The model under review builds one solid part; all positions refer to its coordinate system, in mm. Face numbers are marked on the shaded views. Coordinates: 2 decimals unless noted, no trailing zeros. Loops run counter-clockwise (first coordinate to the right, second up) from the corner with the lowest first, then second, coordinate; pieces in that order, holes last. Notation, with made-up numbers: (43.5, 7) - (99.5, 7) arc R15 cw to (99.5, 19) - close; hole circle Ø10 at (88, 62.25). An arc over 180 degrees is marked (long way). Use a Markdown table: item, result. Add a question column.
1) The part is to be moulded in two halves that separate along X. For the marked faces 1, 2 and 3, say which applies: pulls with the +X half, pulls with the -X half, needs draft (parallel to the pull), parting line crosses it, or undercut.
2) Add section C-C, the plane x = 0. Give the boundary of the cut face in (y, z).
3) Clearance check with flat-ended pins moving along their axes: pin 1 (3 mm diameter, centred on y = -54, z = 26.5, fed in from -X); pin 2 (21.5 mm diameter, centred on y = -37, z = 8, fed in from -X); pin 3 (6.5 mm diameter, centred on x = -6.5, z = 2, fed in from -Y). State where each tip first meets the part, or that it passes through.
4) Add section B-B, the plane z = 1.5. Give the boundary of the cut face in (x, y), and give its area (3 significant figures).
5) Add section D-D, the plane z = 23.5. Give the boundary of the cut face in (x, y), and give its area (3 significant figures).
6) To check wall thickness, follow L1, parallel to X at y = -8, z = -3; L2, parallel to X at y = -95, z = -3.5; L3, parallel to Z at x = 35, y = -8. State the ranges of each line that lie inside material, in increasing order. Write a range as [from, to].
7) Add section A-A, the plane y = -25.5. Give the boundary of the cut face in (x, z), and give its area (3 significant figures).
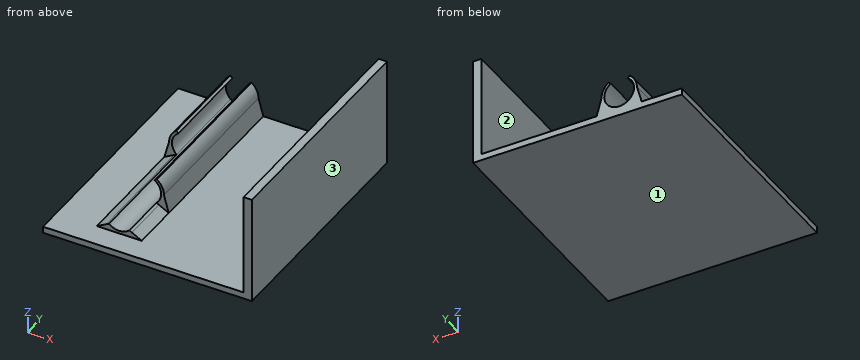
```python
from build123d import *

# Parameters (mm, degrees)
F1_DEPTH = 90
F2_DEPTH = 40
F0_W     = 3.4774128616
F0_H     = 42.5927758359
F3_DEPTH = 100
F4_DEPTH = 70


# Not quite as in the source:
# - a feature names something its author has since deleted; it is built from what else it names


with BuildPart() as f1:
    # F0 (on Front) → F1 (new body)
    with BuildSketch(Plane.XZ):
        with BuildLine():
            ThreePointArc((4.2720749172, -4.5620034965), (0, -6.25), (-4.2720749172, -4.5620034965))
            Line((-4.2720749172, -4.5620034965), (-5.3278356976, -5.1455675625))
            ThreePointArc((-5.3278356976, -5.1455675625), (-2.8939428024, -6.818195789), (0, -7.4069358551))
            ThreePointArc((0, -7.4069358551), (2.8939428024, -6.818195789), (5.3278356976, -5.1455675625))
            Line((5.3278356976, -5.1455675625), (4.2720749172, -4.5620034965))
        make_face()
        with BuildLine():
            Line((9.4190128148, -7.4069358551), (5.3278356976, -5.1455675625))
            ThreePointArc((5.3278356976, -5.1455675625), (2.8939428024, -6.818195789), (0, -7.4069358551))
            Line((0, -7.4069358551), (9.4190128148, -7.4069358551))
        make_face()
        with BuildLine():
            ThreePointArc((0, -7.4069358551), (-2.8939428024, -6.818195789), (-5.3278356976, -5.1455675625))
            Line((-5.3278356976, -5.1455675625), (-9.4190128148, -7.4069358551))
            Line((-9.4190128148, -7.4069358551), (0, -7.4069358551))
        make_face()
        Polygon((9.4190128148, -7.4069358551), (0, -7.4069358551), (0, -10.1), (61.2, -10.1), (61.2, -7.4069358551), (57.7225871384, -7.4069358551), align=None)
    extrude(amount=F1_DEPTH)

    # F0 (on Front) → F2 (join)
    with BuildSketch(Plane.XZ):
        with BuildLine():
            Line((-9.4190128148, -7.4069358551), (-5.3278356976, -5.1455675625))
            ThreePointArc((-5.3278356976, -5.1455675625), (-6.8675190578, -2.7748658979), (-7.4069358551, 0))
            Line((-7.4069358551, 0), (-9.4190128148, -7.4069358551))
        make_face()
        with BuildLine():
            ThreePointArc((-4.2720749172, -4.5620034965), (-6.230456475, 0.4938745919), (-3.5, 5.1780787943))
            Line((-3.5, 5.1780787943), (-4.4709416805, 5.9053686803))
            ThreePointArc((-4.4709416805, 5.9053686803), (-6.6324458912, 3.2974778636), (-7.4069358551, 0))
            ThreePointArc((-7.4069358551, 0), (-6.8675190578, -2.7748658979), (-5.3278356976, -5.1455675625))
            Line((-5.3278356976, -5.1455675625), (-4.2720749172, -4.5620034965))
        make_face()
        with BuildLine():
            ThreePointArc((3.5, 5.1780787943), (6.230456475, 0.4938745919), (4.2720749172, -4.5620034965))
            Line((4.2720749172, -4.5620034965), (5.3278356976, -5.1455675625))
            ThreePointArc((5.3278356976, -5.1455675625), (6.8675190578, -2.7748658979), (7.4069358551, 0))
            ThreePointArc((7.4069358551, 0), (6.6324458912, 3.2974778636), (4.4709416805, 5.9053686803))
            Line((4.4709416805, 5.9053686803), (3.5, 5.1780787943))
        make_face()
        with BuildLine():
            ThreePointArc((7.4069358551, 0), (6.8675190578, -2.7748658979), (5.3278356976, -5.1455675625))
            Line((5.3278356976, -5.1455675625), (9.4190128148, -7.4069358551))
            Line((9.4190128148, -7.4069358551), (7.4069358551, 0))
        make_face()
    extrude(amount=F2_DEPTH)

    # F0 (on Front) → F3 (join)
    with BuildSketch(Plane.XZ):
        Polygon((0, -10.1), (0, -7.4069358551), (-9.4190128148, -7.4069358551), (-26.2554790825, -7.4069358551), (-26.2554790825, -10.1), align=None)
        Polygon((9.4190128148, -7.4069358551), (0, -7.4069358551), (0, -10.1), (61.2, -10.1), (61.2, -7.4069358551), (57.7225871384, -7.4069358551), align=None)
        with Locations((59.4612935692, 13.8894520629)):
            Rectangle(F0_W, F0_H)
    extrude(amount=F3_DEPTH)

    # F0 (on Front) → F4 (join)
    with BuildSketch(Plane.XZ):
        with BuildLine():
            ThreePointArc((3.5, 5.1780787943), (6.230456475, 0.4938745919), (4.2720749172, -4.5620034965))
            Line((4.2720749172, -4.5620034965), (5.3278356976, -5.1455675625))
            ThreePointArc((5.3278356976, -5.1455675625), (6.8675190578, -2.7748658979), (7.4069358551, 0))
            ThreePointArc((7.4069358551, 0), (6.6324458912, 3.2974778636), (4.4709416805, 5.9053686803))
            Line((4.4709416805, 5.9053686803), (3.5, 5.1780787943))
        make_face()
        with BuildLine():
            ThreePointArc((7.4069358551, 0), (6.8675190578, -2.7748658979), (5.3278356976, -5.1455675625))
            Line((5.3278356976, -5.1455675625), (9.4190128148, -7.4069358551))
            Line((9.4190128148, -7.4069358551), (7.4069358551, 0))
        make_face()
    extrude(amount=F4_DEPTH)


solid = f1.part
```
From the geometry:
| question | item | result |
|---|---|---|
| 1 | face 1 | needs draft |
| 1 | face 2 | undercut |
| 1 | face 3 | pulls with the +X half |
| 2 | outline | (-100, -10.1) - (0, -10.1) - (0, -6.25) - (-90, -6.25) - (-90, -7.41) - (-100, -7.41) - close |
| 3 | pin 1 | stops at x = 57.72 |
| 3 | pin 2 | stops at x = -8.15 |
| 3 | pin 3 | stops at y = -40 |
| 4 | outline | (-7.25, -40) - (-6.07, -40) - (-6.07, 0) - (-7.25, 0) - close; (6.07, -70) - (7.25, -70) - (7.25, 0) - (6.07, 0) - close; (57.72, -100) - (61.2, -100) - (61.2, 0) - (57.72, 0) - close |
| 4 | area | 478 mm^2 |
| 5 | outline | (57.72, -100) - (61.2, -100) - (61.2, 0) - (57.72, 0) - close |
| 5 | area | 348 mm^2 |
| 6 | L1 | x = [-8.22, -5.48], [5.48, 8.22], [57.72, 61.2] |
| 6 | L2 | x = [57.72, 61.2] |
| 6 | L3 | z = [-10.1, -7.41] |
| 7 | outline | (-26.26, -10.1) - (61.2, -10.1) - (61.2, 35.19) - (57.72, 35.19) - (57.72, -7.41) - (9.42, -7.41) - (7.41, 0) arc R7.41 ccw to (4.47, 5.91) - (3.5, 5.18) arc R6.25 cw (long way) to (-3.5, 5.18) - (-4.47, 5.91) arc R7.41 ccw to (-7.41, 0) - (-9.42, -7.41) - (-26.26, -7.41) - close |
| 7 | area | 462 mm^2 |
